Verification items for this drawing (mm, ordinates from the low corner). A direction names the side the tool comes from. Give positions to 0.01 mm unless a question says otherwise; leave off trailing zeros. Order: outer loops, then holes, each group sorted by start corner. A loop starts at its lowest first (then second) coordinate and runs counter-clockwise, first axis right, second up. Notation, with made-up numbers: M 57,14.25 L 115,14.25 A31 ccw 115,46.25 Z; hole C 30,-1 d8. An arc over 180 degrees is marked long. Answer as a JSON object with one key per item and string values.
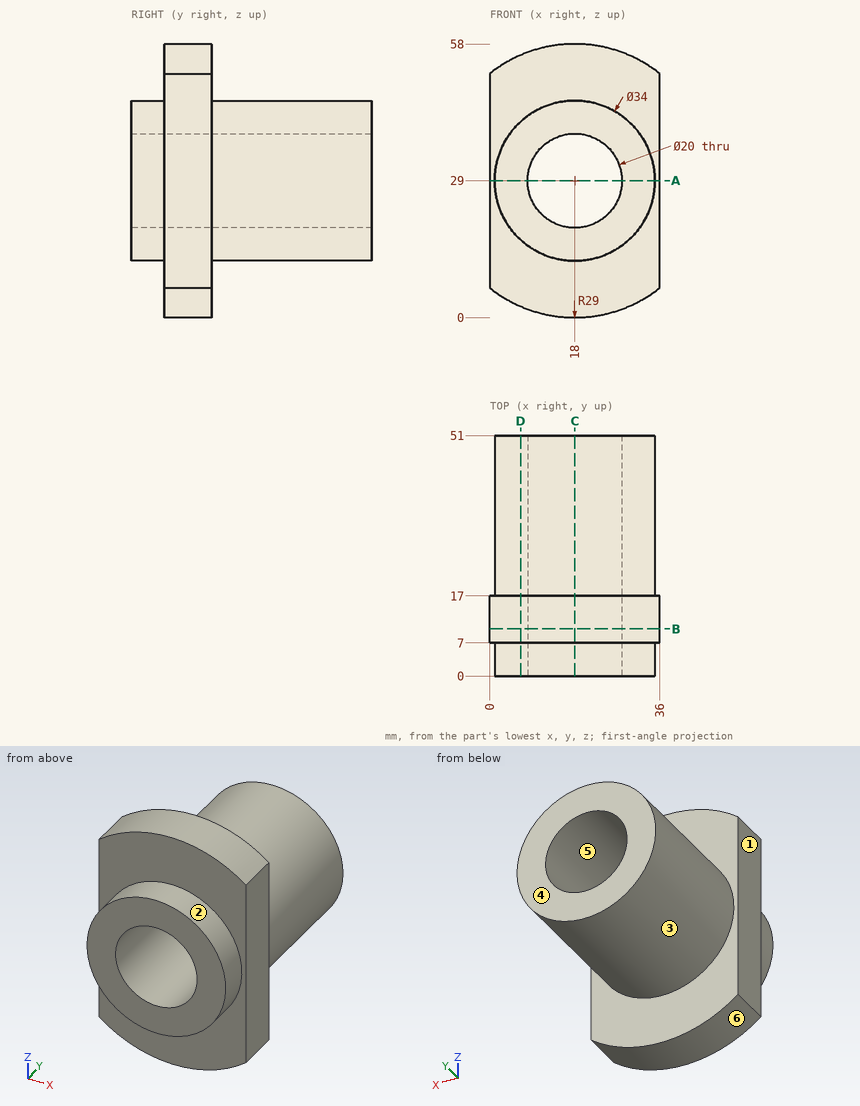
Q1. Tool access check on the marked faces 1, 2 and 3. Record the directions out of +Z, -Z, +X, -X, +Y, -Y that give a thin tool (end or side, any length) a straight path to the whole face; none if there is none.
Resolved:
{"face 1": "+Z, -Z, -X, +Y, -Y", "face 2": "-Y", "face 3": "+Y"}
Q2. Section check D-D on x = 6.5. Record the cut outline in (y, z), then the cut area to 3 significant figures.
Resolved:
{"outline": "M 0,16.48 L 7,16.48 L 7,2.38 L 17,2.38 L 17,16.48 L 51,16.48 L 51,41.52 L 17,41.52 L 17,55.62 L 7,55.62 L 7,41.52 L 0,41.52 Z", "area": "1,560 mm²"}
Q3. Material ranges on L1, parallel to X at y = 37, z = 29; L2, parallel to Z at x = 17.5, y = 16; L3, parallel to Z at x = 18.5, y = 36, recorded low to high.
Resolved:
{"L1": "x = 1 to 8, 28 to 35", "L2": "z = 0 to 19.01, 38.99 to 58", "L3": "z = 12.01 to 19.01, 38.99 to 45.99"}
Q4. Section check C-C on x = 18. Record the cut outline in (y, z).
Resolved:
{"outline": "M 0,12 L 7,12 L 7,0 L 17,0 L 17,12 L 51,12 L 51,19 L 0,19 Z; M 0,39 L 51,39 L 51,46 L 17,46 L 17,58 L 7,58 L 7,46 L 0,46 Z"}
Q5. Gauge pin test, flat ends, axial feed: pin 1 Ø1.5 at (x, y) = (16.5, 42) entering from -Z; pin 2 Ø8 at (x, y) = (8.5, 17) entering from +Z; pin 3 Ø12 at (x, y) = (32, 30) entering from +Z. Record the tip position at first contact, or that the pin passes through.
Resolved:
{"pin 1": "stops at z = 12.02", "pin 2": "stops at z = 57.47", "pin 3": "stops at z = 44"}
Q6. Release check for a two-part mould opening along X. For the marked faces 4, 5 and 6 record: +X half, -X half, draft (parallel to the pull), parting line (faces both ways), or undercut.
Resolved:
{"face 4": "draft", "face 5": "undercut", "face 6": "parting line"}
Q7. Section check B-B on y = 10. Record the cut outline in (x, z).
Resolved:
{"outline": "M 0,6.26 A29 ccw 36,6.26 L 36,51.74 A29 ccw 0,51.74 Z; hole C 18,29 d20"}
Q8. Section check A-A on z = 29. Record the cut outline in (x, y), then the cut area to 3 significant figures.
Resolved:
{"outline": "M 0,7 L 1,7 L 1,0 L 8,0 L 8,51 L 1,51 L 1,17 L 0,17 Z; M 28,0 L 35,0 L 35,7 L 36,7 L 36,17 L 35,17 L 35,51 L 28,51 Z", "area": "734 mm²"}
